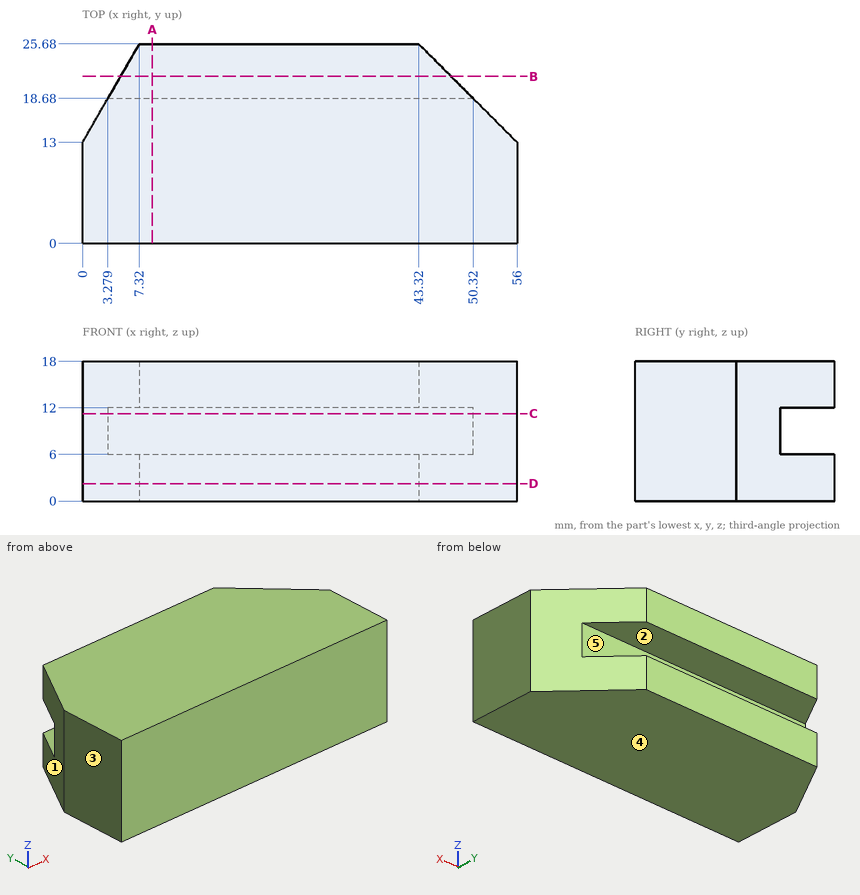
Input: dimensioned drawing with shaded views. Units: mm. Origin: part minimum x, y, z. A direction names the side the tool comes from. Round coordinates to 2 decimals unless told otherwise and drop trailing zeros. Order: outer loops, then holes, each group sorted by start corner. A loop starts at its lowest first (then second) coordinate and runs counter-clockwise, first axis right, second up.
Q1. Section A-A, the plane x = 9. Output: boundary loops of the cut face in (y, z), and give its area (3 significant figures).
Result sheet:
outline: (0, 0) - (25.68, 0) - (25.68, 6) - (18.68, 6) - (18.68, 12) - (25.68, 12) - (25.68, 18) - (0, 18) - close
area: 420 mm2
Q2. Material intervals for probe 1 along Z at (x, y) = (10.5, 21); probe 2 along Y at (x, z) = (21, 6.5); probe 3 along X at (y, z) = (14.5, 6.75) (1 decimal), sorted ascending.
Result sheet:
probe 1: z = 0 to 6, 12 to 18
probe 2: y = 0 to 18.68
probe 3: x = 0.9 to 54.5
Q3. Mould query, pull axis Z, two halves, no side actions, for the marked faces 3, 4 and 5. Classes: released by +Z, released by -Z, zero draft, split by the parting line, or undercut.
Result sheet:
face 3: zero draft
face 4: released by -Z
face 5: undercut
Q4. Section D-D, the plane z = 2.25. Output: boundary loops of the cut face in (x, y).
Result sheet:
outline: (0, 0) - (56, 0) - (56, 13) - (43.32, 25.68) - (7.32, 25.68) - (0, 13) - close
Q5. Section C-C, the plane z = 11.25. Output: boundary loops of the cut face in (x, y), and give its area (3 significant figures).
Result sheet:
outline: (0, 0) - (56, 0) - (56, 13) - (50.32, 18.68) - (3.28, 18.68) - (0, 13) - close
area: 1,020 mm2
Q6. Access query for the marked faces 1 and 2. Directions: +Z, -Z, +X, -X, +Y, -Y. A direction counts if a zero-diameter tool reaches every point of the face in a straight line with its end or side. Return the directions, or none.
Result sheet:
face 1: +Z, -Z, -X, +Y
face 2: +X, -X, +Y
Q7. Section B-B, the plane y = 21.5. Output: boundary loops of the cut face in (x, z), and give its area (3 significant figures).
Result sheet:
outline: (4.91, 0) - (47.5, 0) - (47.5, 6) - (4.91, 6) - close; (4.91, 12) - (47.5, 12) - (47.5, 18) - (4.91, 18) - close
area: 511 mm2
